from build123d import *

# Parameters (mm, degrees)
F0_R     = 10.795
F1_DEPTH = 20.32
F3_DEPTH = 37.415268


with BuildPart() as f1:
    # F0 (on Front) → F1 (new body)
    with BuildSketch(Plane.XZ):
        with BuildLine():
            ThreePointArc((-5.08, 12.7), (-3.12545, 6.11582), (0, 0))
            Line((0, 0), (134.62, 0))
            ThreePointArc((134.62, 0), (135.239562, 3.067997), (132.842, 5.08))
            ThreePointArc((132.842, 5.08), (117.272541, 6.983954), (101.6, 7.62))
            ThreePointArc((101.6, 7.62), (62.641831, 14.148311), (27.94, 33.02))
            ThreePointArc((27.94, 33.02), (4.360893, 34.347299), (-5.08, 12.7))
        make_face()
        with Locations((17.78, 12.7)):
            Circle(F0_R, mode=Mode.SUBTRACT)
    extrude(amount=F1_DEPTH)

    # F2 (on face) → F3 (cut, through all)
    with BuildSketch(Plane(origin=(0, 0, 0), x_dir=(1, 0, 0), z_dir=(0, 0, -1))):
        with BuildLine():
            ThreePointArc((17.78, 6.35), (20.474077, 7.465923), (21.59, 10.16))
            ThreePointArc((21.59, 10.16), (20.474077, 12.854077), (17.78, 13.97))
            Line((17.78, 13.97), (17.78, 6.35))
        make_face()
        with BuildLine():
            Line((17.78, 6.35), (17.78, 13.97))
            ThreePointArc((17.78, 13.97), (13.97, 10.16), (17.78, 6.35))
        make_face()
    extrude(amount=-F3_DEPTH, mode=Mode.SUBTRACT)


solid = f1.part
CAD build for the part. Positions are in the model's coordinates, mm. Give positions to 0.01 mm unless a question says otherwise; leave off trailing zeros. Order: outer loops, then holes, each group sorted by start corner. A loop starts at its lowest first (then second) coordinate and runs counter-clockwise, first axis right, second up. Notation, with made-up numbers: (60.25, 37.25) - (76.25, 37.25) arc R34 cw to (76.25, 71.25) - close; hole circle Ø7 at (-22, 82). An arc over 180 degrees is marked (long way). Write each question's results on one line, items separated by ' | '.
1. Pull direction X, two halves, no side cores. Call faces 1 (the face through (63.167, -10.018, 13.968)), 2 (the face through (66, -10, 0)), 3 (the face through (27.752, -10.018, 8.565)): released by +X, released by -X, zero draft, split by the parting line, or undercut.
Calculated:
face 1: released by +X | face 2: zero draft | face 3: undercut
2. Pin check, flat tips, straight feed: pin 1 (1 mm diameter, centred on x = 78, y = -6, fed in from +Z); pin 2 (4 mm diameter, centred on x = 12, y = -5, fed in from +Z); pin 3 (12 mm diameter, centred on x = 98.5, y = -9, fed in from +Z); pin 4 (19.5 mm diameter, centred on x = 17.78, z = 12.7, fed in from +Y). Stop position of each tip, or through.
Calculated:
pin 1: stops at z = 10.08 | pin 2: stops at z = 37.38 | pin 3: stops at z = 7.97 | pin 4: passes through
3. Saw through at C-C on z = 26.5. List the corners of the cut face in (x, y), and give its area (3 significant figures).
Calculated:
outline: (-3.03, -20.32) - (37.13, -20.32) - (37.13, 0) - (-3.03, 0) - close; hole (17.78, -6.35) arc R3.81 ccw (long way) to (21.59, -10.16) arc R3.81 ccw to start | area: 770 mm2
4. Probe L1, parallel to X at y = -7, z = 24; L2, parallel to X at y = -13.75, z = 18; L3, parallel to Z at x = 126.5, y = -8. List the from-to ranges inside material, lowest first. Write a range as from..to.
Calculated:
L1: x = -4.16..15.65, 19.91..41.21 | L2: x = -5.44..8.38, 27.18..52.88 | L3: z = 0..6.01
5. Saw through at D-D on x = 91.5. List the corners of the cut face in (y, z).
Calculated:
outline: (-20.32, 0) - (0, 0) - (0, 8.05) - (-20.32, 8.05) - close
6. Saw through at B-B on y = -11.75. List the corners of the cut face in (x, z) (3 decimals).
Calculated:
outline: (-5.08, 12.7) arc R37.405 ccw to (0, 0) - (14.318, 0) - (14.318, 2.475) arc R10.795 cw to (14.318, 22.925) - (14.318, 37.396) arc R20.675 ccw to start; (21.242, 0) - (134.62, 0) arc R3.065 ccw to (132.842, 5.08) arc R193.408 ccw to (101.6, 7.62) arc R119.507 cw to (27.94, 33.02) arc R20.675 ccw to (21.242, 36.511) - (21.242, 22.925) arc R10.795 cw to (21.242, 2.475) - close
7. Saw through at A-A on z = 17.5. List the corners of the cut face in (x, y).
Calculated:
outline: (-5.46, -20.32) - (8.11, -20.32) - (8.11, 0) - (-5.46, 0) - close; (27.45, -20.32) - (54.02, -20.32) - (54.02, 0) - (27.45, 0) - close
